Read the model definition and answer for the solid it produces. Units are mm, in the model's axes. A direction names the side the tool comes from. Give positions to 0.01 mm unless a question says otherwise; leave off trailing zeros. Order: outer loops, then holes, each group sorted by start corner. A loop starts at its lowest first (then second) coordinate and runs counter-clockwise, first axis right, second up. Notation, with made-up numbers: (4, 50.5) - (46, 50.5) arc R15 ccw to (46, 72.5) - close; hole circle Ø5 at (24.25, -3). An arc over 180 degrees is marked (long way). Write each question's results on one line, items separated by ' | '. Start each with the question number.
Q1. Flat-ended cylindrical pins translate along their axes: P1, Ø14.5, axis at x = -60, y = 0, coming from the +Z side; P2, Ø6, axis at x = 5, z = 63.5, coming from the +Y side; P3, Ø12, axis at x = -59, z = 43, coming from the +Y side; P4, Ø10, axis at x = -16.5, z = 38.5, coming from the -Y side. Find the tip coordinate at first contact, or state that the pin passes through.
Q2. Find section C-C on y = 6. Give the vertices of the cut face in (x, z), and give its area (3 significant figures).
Q3. Find section D-D on x = -81.5. Give the vertices of the cut face in (y, z), and give its area (3 significant figures).
Q4. Find the intervals of material crossed by line 1 along Y through (x, z) = (0, 68); line 2 along Z through (x, y) = (5, -22); line 3 along Y through (x, z) = (6, 48.5), in increasing order. Write a range as from..to.
Q5. Find section A-A on x = 0. Give the vertices of the cut face in (y, z), and give its area (3 significant figures).
Q6. Find section B-B on z = 53. Give the vertices of the cut face in (x, y), and give its area (3 significant figures).
Q7. A tool of negligible diameter and unlimited length cuts with its end or side. For faces 4 (the face through (-31, 0, -3)), 5 (the face through (-31, 0, 0)), from which of +Z, -Z, +X, -X, +Y, -Y can it reach the whole face along a straight path? Write none if from no direction.
Q8. For a pull along Y with two mould halves and no side action, classify faces 1 (the face through (-2.17, -9.76, 36.98)), 2 (the face through (-60, 8.2, 75)), 3 (the face through (0, 0, 65)) as +Y half, -Y half, draft (parallel to the pull), parting line (faces both ways), or undercut.
from build123d import *

# Parameters (mm, degrees)
F0_W     = 120
F0_H     = 60
F0_R     = 10
F1_DEPTH = 3
F2_DEPTH = 75
F3_R     = 8
F4_DEPTH = 10


with BuildPart() as f1:
    # F0 (on Top) → F1 (new body)
    with BuildSketch(Plane.XY):
        with Locations((-30, 0)):
            Rectangle(F0_W, F0_H)
        with Locations((-60, 0)):
            Circle(F0_R, mode=Mode.SUBTRACT)
        Circle(F0_R, mode=Mode.SUBTRACT)
        with Locations((-60, 0)):
            Circle(F0_R)
        Circle(F0_R)
    extrude(amount=-F1_DEPTH)

    # F0 (on Top) → F2 (join)
    with BuildSketch(Plane.XY):
        with Locations((-60, 0)):
            Circle(F0_R)
        Circle(F0_R)
    extrude(amount=F2_DEPTH)

    # F3 (on face) → F4 (cut)
    with BuildSketch(Plane.XY.offset(75)):
        with Locations((-60, 0)):
            Circle(F3_R)
        Circle(F3_R)
    extrude(amount=-F4_DEPTH, mode=Mode.SUBTRACT)


solid = f1.part
Working result:
1) P1: z = 65 | P2: y = 9.8 | P3: y = 10 | P4: through
2) outline: (-90, -3) - (30, -3) - (30, 0) - (8, 0) - (8, 75) - (5.29, 75) - (5.29, 65) - (-5.29, 65) - (-5.29, 75) - (-8, 75) - (-8, 0) - (-52, 0) - (-52, 75) - (-54.71, 75) - (-54.71, 65) - (-65.29, 65) - (-65.29, 75) - (-68, 75) - (-68, 0) - (-90, 0) - close | area: 2,550 mm²
3) outline: (-30, -3) - (30, -3) - (30, 0) - (-30, 0) - close | area: 180 mm²
4) line 1: -10..-8, 8..10 | line 2: -3..0 | line 3: -8..8
5) outline: (-30, -3) - (30, -3) - (30, 0) - (10, 0) - (10, 75) - (8, 75) - (8, 65) - (-8, 65) - (-8, 75) - (-10, 75) - (-10, 0) - (-30, 0) - close | area: 1,520 mm²
6) outline: circle Ø20 at (-60, 0); circle Ø20 at (0, 0) | area: 628 mm²
7) face 4: -Z, +X, -X, +Y, -Y | face 5: +Z
8) face 1: parting line | face 2: draft | face 3: undercut
